```python
from build123d import *

# Parameters (mm, degrees)
F0_R     = 1.6050327283
F0_W     = 2.2255629301
F0_H     = 2
F0_W_2   = 1.7703343183
F0_W_3   = 2.1244008094
F1_DEPTH = 0.9
F3_W     = 37.4999957172
F3_H     = 3.8157890567
F3_H_2   = 3.0263150231
F3_H_3   = 2.8947356249
F4_DEPTH = 0.9


with BuildPart() as f1:
    # F0 (on Top) → F1 (new body)
    with BuildSketch(Plane.XY):
        Polygon((-56.3586414655, -11.5456737704), (-60.406261386, -29.879005636), (29.593738614, -29.879005636), (56.3437383481, -43.4597830152), (66.3437383481, -43.4597830152), (66.3437383481, 10.120994364), (-13.6562616519, 10.120994364), (-43.9776898843, 5.1209918552), align=None)
        Polygon((-51.9591234624, -27.8780460358), (-51.9591234624, -25.8780460358), (-46.79986462, -25.8780460358), (-44.5743016899, -25.8780460358), (-38.9092303813, -25.8780460358), (-37.138896063, -25.8780460358), (-30.8162737638, -25.8780460358), (-28.6918729544, -25.8780460358), (-22.3186686635, -25.8780460358), (-22.3186686635, -27.8780460358), (-28.6918729544, -27.8780460358), (-30.8162737638, -27.8780460358), (-37.138896063, -27.8780460358), (-38.9092303813, -27.8780460358), (-44.5743016899, -27.8780460358), (-46.79986462, -27.8780460358), align=None, mode=Mode.SUBTRACT)
        with Locations((59.4792403281, -39.1563028097)):
            Circle(F0_R, mode=Mode.SUBTRACT)
        with BuildLine():
            Line((-16.5355233229, -2.2097615232), (-14.5946062265, -2.2097615232))
            Line((-14.5946062265, -2.2097615232), (-14.5946062265, -13.0145655474))
            add(Edge.make_bspline(
                [(-14.5946062265, -13.0145655474), (-14.5946062265, -15.8729406309), (-16.3198658677, -17.5068199945)],
                knots=[0, 0, 0, 1, 1, 1], degree=2))
            add(Edge.make_bspline(
                [(-16.3198658677, -17.5068199945), (-18.045125509, -19.1406993581), (-21.06067467, -19.1406993581)],
                knots=[0, 0, 0, 1, 1, 1], degree=2))
            add(Edge.make_bspline(
                [(-21.06067467, -19.1406993581), (-24.076223831, -19.1406993581), (-25.7265516446, -17.4940267556)],
                knots=[0, 0, 0, 1, 1, 1], degree=2))
            add(Edge.make_bspline(
                [(-25.7265516446, -17.4940267556), (-27.3768794581, -15.8473541532), (-27.3768794581, -12.9707030141)],
                knots=[0, 0, 0, 1, 1, 1], degree=2))
            Line((-27.3768794581, -12.9707030141), (-27.3768794581, -2.2097615232))
            Line((-27.3768794581, -2.2097615232), (-25.4323071507, -2.2097615232))
            Line((-25.4323071507, -2.2097615232), (-25.4323071507, -13.105945825))
            add(Edge.make_bspline(
                [(-25.4323071507, -13.105945825), (-25.4323071507, -15.1967265766), (-24.2900536806, -16.3170487801)],
                knots=[0, 0, 0, 1, 1, 1], degree=2))
            add(Edge.make_bspline(
                [(-24.2900536806, -16.3170487801), (-23.1478002105, -17.4373709835), (-20.9327422813, -17.4373709835)],
                knots=[0, 0, 0, 1, 1, 1], degree=2))
            add(Edge.make_bspline(
                [(-20.9327422813, -17.4373709835), (-18.8200302631, -17.4373709835), (-17.677776793, -16.3115659634)],
                knots=[0, 0, 0, 1, 1, 1], degree=2))
            add(Edge.make_bspline(
                [(-17.677776793, -16.3115659634), (-16.5355233229, -15.1857609433), (-16.5355233229, -13.0840145583)],
                knots=[0, 0, 0, 1, 1, 1], degree=2))
            Line((-16.5355233229, -13.0840145583), (-16.5355233229, -2.2097615232))
        make_face(mode=Mode.SUBTRACT)
        with BuildLine():
            Line((-4.7474675117, -11.9655199604), (-8.2345389051, -11.9655199604))
            Line((-8.2345389051, -11.9655199604), (-8.2345389051, -18.9104210585))
            Line((-8.2345389051, -18.9104210585), (-10.1754560015, -18.9104210585))
            Line((-10.1754560015, -18.9104210585), (-10.1754560015, -2.2097615232))
            Line((-10.1754560015, -2.2097615232), (-5.5954764878, -2.2097615232))
            add(Edge.make_bspline(
                [(-5.5954764878, -2.2097615232), (-2.5214439492, -2.2097615232), (-1.0538766908, -3.3867394987)],
                knots=[0, 0, 0, 1, 1, 1], degree=2))
            add(Edge.make_bspline(
                [(-1.0538766908, -3.3867394987), (0.4136905676, -4.5637174743), (0.4136905676, -6.9286390588)],
                knots=[0, 0, 0, 1, 1, 1], degree=2))
            add(Edge.make_bspline(
                [(0.4136905676, -6.9286390588), (0.4136905676, -10.2402603192), (-2.9454484373, -11.4062726615)],
                knots=[0, 0, 0, 1, 1, 1], degree=2))
            Line((-2.9454484373, -11.4062726615), (1.5906685431, -18.9104210585))
            Line((1.5906685431, -18.9104210585), (-0.7048040303, -18.9104210585))
            Line((-0.7048040303, -18.9104210585), (-4.7474675117, -11.9655199604))
        make_face(mode=Mode.SUBTRACT)
        with BuildLine():
            add(Edge.make_bspline(
                [(15.2282611731, -4.5966143742), (13.33120661, -3.7083980759), (11.4341520469, -3.7083980759)],
                knots=[0, 0, 0, 1, 1, 1], degree=2))
            add(Edge.make_bspline(
                [(11.4341520469, -3.7083980759), (8.6817780854, -3.7083980759), (7.0881060439, -5.5414864447)],
                knots=[0, 0, 0, 1, 1, 1], degree=2))
            add(Edge.make_bspline(
                [(7.0881060439, -5.5414864447), (5.4944340025, -7.3745748135), (5.4944340025, -10.5619188964)],
                knots=[0, 0, 0, 1, 1, 1], degree=2))
            add(Edge.make_bspline(
                [(5.4944340025, -10.5619188964), (5.4944340025, -13.8369880458), (7.0314502718, -15.6262138814)],
                knots=[0, 0, 0, 1, 1, 1], degree=2))
            add(Edge.make_bspline(
                [(7.0314502718, -15.6262138814), (8.5684665412, -17.4154397169), (11.4122207803, -17.4154397169)],
                knots=[0, 0, 0, 1, 1, 1], degree=2))
            add(Edge.make_bspline(
                [(11.4122207803, -17.4154397169), (13.1594116881, -17.4154397169), (15.400056095, -16.786743407)],
                knots=[0, 0, 0, 1, 1, 1], degree=2))
            Line((15.400056095, -16.786743407), (15.400056095, -18.4864165704))
            add(Edge.make_bspline(
                [(15.400056095, -18.4864165704), (13.6638308205, -19.1406993581), (11.1161486808, -19.1406993581)],
                knots=[0, 0, 0, 1, 1, 1], degree=2))
            add(Edge.make_bspline(
                [(11.1161486808, -19.1406993581), (7.4280406766, -19.1406993581), (5.4231573859, -16.9000549512)],
                knots=[0, 0, 0, 1, 1, 1], degree=2))
            add(Edge.make_bspline(
                [(5.4231573859, -16.9000549512), (3.4182740953, -14.6594105443), (3.4182740953, -10.5363324187)],
                knots=[0, 0, 0, 1, 1, 1], degree=2))
            add(Edge.make_bspline(
                [(3.4182740953, -10.5363324187), (3.4182740953, -7.9557533791), (4.3832498268, -6.0148362827)],
                knots=[0, 0, 0, 1, 1, 1], degree=2))
            add(Edge.make_bspline(
                [(4.3832498268, -6.0148362827), (5.3482255583, -4.0739191863), (7.1703482938, -3.0230459939)],
                knots=[0, 0, 0, 1, 1, 1], degree=2))
            add(Edge.make_bspline(
                [(7.1703482938, -3.0230459939), (8.9924710293, -1.9721728014), (11.4597385246, -1.9721728014)],
                knots=[0, 0, 0, 1, 1, 1], degree=2))
            add(Edge.make_bspline(
                [(11.4597385246, -1.9721728014), (14.0841800975, -1.9721728014), (16.0506836716, -2.9298381107)],
                knots=[0, 0, 0, 1, 1, 1], degree=2))
            Line((16.0506836716, -2.9298381107), (15.2282611731, -4.5966143742))
        make_face(mode=Mode.SUBTRACT)
        with Locations((-45.6870831549, -26.8780460358)):
            Rectangle(F0_W, F0_H)
        with Locations((-38.0240632221, -26.8780460358)):
            Rectangle(F0_W_2, F0_H)
        with Locations((-29.7540733591, -26.8780460358)):
            Rectangle(F0_W_3, F0_H)
    extrude(amount=F1_DEPTH)

    # F3 (on face) → F4 (cut, through all)
    with BuildSketch(Plane.XY.offset(0.9)):
        with Locations((40.5594706535, -1.704487608)):
            Rectangle(F3_W, F3_H)
        with Locations((40.5594706535, -18.0202752728)):
            Rectangle(F3_W, F3_H_2)
        with Locations((40.5594706535, -10.0597499488)):
            Rectangle(F3_W, F3_H_3)
    extrude(amount=-F4_DEPTH, mode=Mode.SUBTRACT)


solid = f1.part
```
Could you check a few things on this model? Use its own coordinates, in mm. A direction names the side the tool comes from. Coordinates: 2 decimals unless noted, no trailing zeros. Write each loop counter-clockwise with the first axis right and the second up, starting at its lowest first coordinate (ties: lowest second). Pieces come first, ordered by that corner, then holes. Notation, with made-up numbers: (4.5, -31.75) - (45.5, -31.75) arc R31 cw to (45.5, 4.25) - close; hole circle Ø4 at (-38, 87.25). An arc over 180 degrees is marked (long way). Use a Markdown table: item, result.
Q1. Which directions (+Z, -Z, +X, -X, +Y, -Y) give clear straight access to the entire face, cutting with the end or side of a thin tool? Please do faces 1 (the flat face through (-2.698, -15.487, 0.444)), 2 (the flat face through (-28.605, 7.656, 0.444)).
Geometry check:
| item | result |
|---|---|
| face 1 | +Z, -Z |
| face 2 | +Z, -Z, -X, +Y |
Q2. Imagine slicing it at D-D (y = -36). List the corners of the cut face in (x, z) for me, and give its area (3 significant figures).
Geometry check:
| item | result |
|---|---|
| outline | (41.65, 0) - (66.34, 0) - (66.34, 0.9) - (41.65, 0.9) - close |
| area | 22.2 mm2 |
Q3. Please list where these lines run through material, in increasing order: L1, parallel to Y at x = 22, z = 0.15; L2, parallel to X at y = -26, z = 0.75; L3, parallel to X at y = -27.5, z = 0.4.
Geometry check:
| item | result |
|---|---|
| L1 | y = -29.88 to -19.53, -16.51 to -11.51, -8.61 to -3.61, 0.2 to 10.12 |
| L2 | x = -59.55 to -51.96, -46.8 to -44.57, -38.91 to -37.14, -30.82 to -28.69, -22.32 to 66.34 |
| L3 | x = -59.88 to -51.96, -46.8 to -44.57, -38.91 to -37.14, -30.82 to -28.69, -22.32 to 66.34 |
Q4. Imagine slicing it at B-B (y = -10). Count the separate pieces of the cut face and the enclosed holes in it, and give its area (3 significant figures).
Geometry check:
| item | result |
|---|---|
| separate pieces | 6 |
| enclosed holes | 0 |
| area | 61.7 mm2 |
Q5. Imagine slicing it at A-A (x = 43). List the corners of the cut face in (y, z) for me.
Geometry check:
| item | result |
|---|---|
| outline | (-36.69, 0) - (-19.53, 0) - (-19.53, 0.9) - (-36.69, 0.9) - close; (-16.51, 0) - (-11.51, 0) - (-11.51, 0.9) - (-16.51, 0.9) - close; (-8.61, 0) - (-3.61, 0) - (-3.61, 0.9) - (-8.61, 0.9) - close; (0.2, 0) - (10.12, 0) - (10.12, 0.9) - (0.2, 0.9) - close |
Q6. I'm going to push flat-ended pins straight in: pin 1 Ø8 at (x, y) = (-7.5, -36.5) entering from +Z; pin 2 Ø5 at (x, y) = (-17.5, -22.5) entering from -Z. Where does each tip first touch, or does it pass through?
Geometry check:
| item | result |
|---|---|
| pin 1 | passes through |
| pin 2 | stops at z = 0 |
Q7. Thinking about a two-plate mould opening in Y: for faces 3 (the flat face through (42.781, -36.574, 0.444)), 4 (the cylindrical face through (58.206, -40.133, 0.444)), 5 (the flat face through (2, -10, 0)), which applies, +Y half, -Y half, draft (parallel to the pull), parting line (faces both ways), or undercut?
Geometry check:
| item | result |
|---|---|
| face 3 | -Y half |
| face 4 | undercut |
| face 5 | draft |
